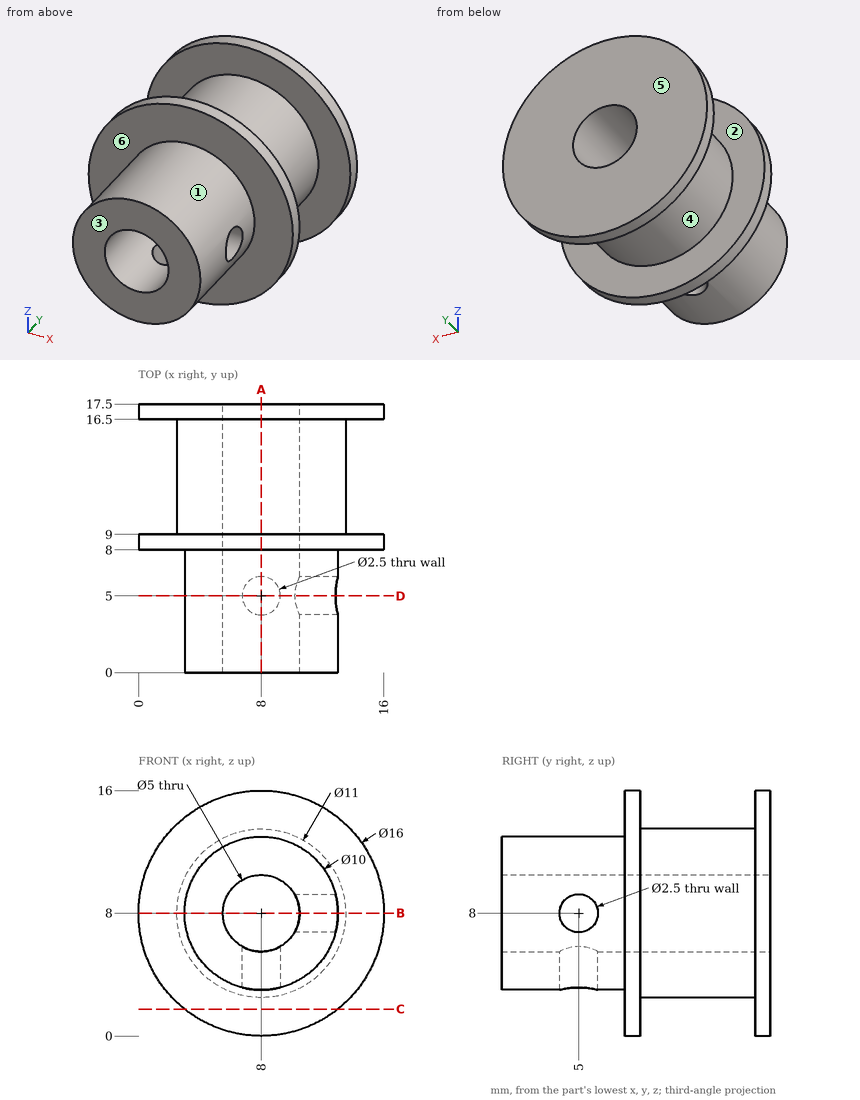
Can you work these out from the drawing? Everything is in mm from the part's minimum corner. A direction names the side the tool comes from. Coordinates: 2 decimals unless noted, no trailing zeros. Order: outer loops, then holes, each group sorted by start corner. A loop starts at its lowest first (then second) coordinate and runs counter-clockwise, first axis right, second up. Notation, with made-up numbers: (27, -36) -> (78, -36) arc R32 ccw to (78, -4) -> close; hole circle Ø3 at (-4.75, 68). An arc over 180 degrees is marked (long way). Return JSON: item names as keys, results as strings.
1) I'm going to push flat-ended pins straight in: P1, Ø8, axis at x = 13.5, y = 9.5, coming from the +Z side; P2, Ø2, axis at x = 8, y = 5, coming from the +Z side; P3, Ø4, axis at x = 4.5, y = 5, coming from the +Z side; P4, Ø3, axis at x = 8, z = 8, coming from the +Y side. Where does each tip first touch, or does it pass through?
Conclusion:
{"P1": "stops at z = 15.85", "P2": "stops at z = 13", "P3": "stops at z = 12.77", "P4": "passes through"}
2) On a 3-axis mill with a long thin cutter (end or side, diameter ignored), from which of +Z, -Z, +X, -X, +Y, -Y can I reach the whole of each face in a straight line? I mean the marked faces 1, 2 and 3. Say none if no direction works.
Conclusion:
{"face 1": "-Y", "face 2": "none", "face 3": "+Z, -Z, +X, -X, -Y"}
3) If we section it at D-D on y = 5: List the corners of the cut face in (x, z) for me.
Conclusion:
{"outline": "(6.75, 3.16) -> (6.75, 5.83) arc R2.5 cw (long way) to (10.17, 9.25) -> (12.84, 9.25) arc R5 ccw (long way) to start; (9.25, 3.16) arc R5 ccw to (12.84, 6.75) -> (10.17, 6.75) arc R2.5 cw to (9.25, 5.83) -> close"}
4) If I drill on probe 1 along Y at (x, z) = (2.5, 2.25); probe 2 along Y at (x, z) = (8, 4.6); probe 3 along X at (y, z) = (13.5, 8), over which ranges is the centre line in solid material (lowest first)?
Conclusion:
{"probe 1": "y = 8 to 9, 16.5 to 17.5", "probe 2": "y = 0 to 3.75, 6.25 to 17.5", "probe 3": "x = 2.5 to 5.5, 10.5 to 13.5"}
5) If we section it at B-B on z = 8: List the corners of the cut face in (x, y) for me, plus the area to 3 significant figures.
Conclusion:
{"outline": "(0, 8) -> (3, 8) -> (3, 0) -> (5.5, 0) -> (5.5, 17.5) -> (0, 17.5) -> (0, 16.5) -> (2.5, 16.5) -> (2.5, 9) -> (0, 9) -> close; (10.5, 0) -> (13, 0) -> (13, 3.75) -> (10.5, 3.75) -> close; (10.5, 6.25) -> (13, 6.25) -> (13, 8) -> (16, 8) -> (16, 9) -> (13.5, 9) -> (13.5, 16.5) -> (16, 16.5) -> (16, 17.5) -> (10.5, 17.5) -> close", "area": "101 mm²"}
6) Thinking about a two-plate mould opening in Y: for the marked faces 4, 5 and 6, which applies, +Y half, -Y half, draft (parallel to the pull), parting line (faces both ways), or undercut?
Conclusion:
{"face 4": "undercut", "face 5": "+Y half", "face 6": "-Y half"}
7) If we section it at C-C on z = 1.75: List the corners of the cut face in (x, y) for me, plus the area to 3 significant figures.
Conclusion:
{"outline": "(3.01, 8) -> (12.99, 8) -> (12.99, 9) -> (3.01, 9) -> close; (3.01, 16.5) -> (12.99, 16.5) -> (12.99, 17.5) -> (3.01, 17.5) -> close", "area": "20.0 mm²"}
8) If we section it at A-A on x = 8: List the corners of the cut face in (y, z) for me.
Conclusion:
{"outline": "(0, 3) -> (3.75, 3) -> (3.75, 5.5) -> (0, 5.5) -> close; (0, 10.5) -> (17.5, 10.5) -> (17.5, 16) -> (16.5, 16) -> (16.5, 13.5) -> (9, 13.5) -> (9, 16) -> (8, 16) -> (8, 13) -> (0, 13) -> close; (6.25, 3) -> (8, 3) -> (8, 0) -> (9, 0) -> (9, 2.5) -> (16.5, 2.5) -> (16.5, 0) -> (17.5, 0) -> (17.5, 5.5) -> (6.25, 5.5) -> close"}
